Geometry check sheet. Reference: the model listing, model coordinates, mm. A direction names the side the tool comes from. Round coordinates to 2 decimals unless told otherwise and drop trailing zeros. Write each loop counter-clockwise with the first axis right and the second up, starting at its lowest first coordinate (ties: lowest second). Pieces come first, ordered by that corner, then holes. Notation, with made-up numbers: M 16.5,36 L 39.5,36 A34 cw 39.5,68 Z; hole C -28.75,80 d4. An arc over 180 degrees is marked long. Answer in a Markdown table with one row per item. Add a question column.
from build123d import *

# Parameters (mm, degrees)
SKETCH1_R                 = 1.778
BOSS_EXTRUDE1_DEPTH       = 6.35
FILLET1_R                 = 1.27
F_6_32_TAPPED_HOLE1_D     = 2.7051
F_6_CLEARANCE_HOLE1_D     = 3.6576
F_6_CLEARANCE_HOLE1_DEPTH = 3.175
F_6_CLEARANCE_HOLE1_TIP   = 1.0988539


with BuildPart() as part:
    # Sketch1 → Boss-Extrude1 (new body)
    with BuildSketch(Plane.XY):
        with BuildLine():
            Line((-5.04, 40.467867395), (-5.04, 31.75))
            Line((-5.04, 31.75), (-5.04, 5.617641854))
            ThreePointArc((-5.04, 5.617641854), (-5.205917611, 4.175551358), (-5.695, 2.808820927))
            ThreePointArc((-5.695, 2.808820927), (1.46358213, -6.179031263), (3.83, 5.064938302))
            ThreePointArc((3.83, 5.064938302), (1.974799916, 7.301272707), (1.31, 10.129876603))
            Line((1.31, 10.129876603), (1.31, 23.320498235))
            ThreePointArc((1.31, 23.320498235), (1.853099889, 25.890013969), (3.389499561, 28.020000975))
            ThreePointArc((3.389499561, 28.020000975), (4.60894119, 29.710573339), (5.04, 31.75))
            Line((5.04, 31.75), (5.04, 40.467867395))
            Line((5.04, 40.467867395), (2.5, 40.467867395))
            Line((2.5, 40.467867395), (2.5, 31.75))
            ThreePointArc((2.5, 31.75), (-1.456880228, 29.718375035), (-0.802, 34.117867395))
            Line((-0.802, 34.117867395), (-0.802, 40.467867395))
            Line((-0.802, 40.467867395), (-5.04, 40.467867395))
        make_face()
        Circle(SKETCH1_R, mode=Mode.SUBTRACT)
    extrude(amount=BOSS_EXTRUDE1_DEPTH)

    # Fillet1
    fillet1_edges = [part.edges().sort_by_distance(p)[0] for p in [
        (-5.04, 40.467867395, 3.175),
    ]]
    fillet(fillet1_edges, radius=FILLET1_R)

    # #6-32 Tapped Hole1 (through all)
    with Locations(Plane.ZY.offset(5.04)):
        with Locations((3.175, 37.292867395)):
            Hole(F_6_32_TAPPED_HOLE1_D / 2)

    # #6 Clearance Hole1
    with Locations(Plane(origin=(5.04, 37.292867395, 3.175), x_dir=(0, 1, 0), z_dir=(1, 0, 0))):
        with Locations((0, 0)):
            Hole(F_6_CLEARANCE_HOLE1_D / 2, depth=F_6_CLEARANCE_HOLE1_DEPTH)
            with Locations((0, 0, -(F_6_CLEARANCE_HOLE1_DEPTH + F_6_CLEARANCE_HOLE1_TIP / 2))):  # 118° drill point
                Cone(0, F_6_CLEARANCE_HOLE1_D / 2, F_6_CLEARANCE_HOLE1_TIP, mode=Mode.SUBTRACT)


solid = part.part
Item 1: Gauge pin test, flat ends, axial feed: pin 1 Ø3 at (y, z) = (38.5, 3.5) entering from +X; pin 2 Ø2 at (y, z) = (34, 4) entering from -X; pin 3 Ø3 at (x, y) = (0, 0) entering from -Z. Record the tip position at first contact, or that the pin passes through.
Item 2: Scan lines: probe 1 along X at (y, z) = (31.75, 2); probe 2 along Y at (x, z) = (0, 1.5); probe 3 along Y at (x, z) = (-1, 2.75). Record each from-to range of solid material in increasing order. Write a range as from..to.
Item 3: Section check D-D, the plane y = 17. Record the boundary of the cut face in (x, z).
Item 4: Mould release check, pull along Y, two halves, no side actions. Record for faces 6 (the cylindrical face through (4.597, 29.684, 3.131)), 7 (the cylindrical face through (-4.678, 40.086, 3.219)), 8 (the flat face through (5.04, 35, 3)): +Y half, -Y half, draft (parallel to the pull), parting line (faces both ways), or undercut.
Item 5: Section check A-A, the plane y = 0. Record the boundary of the cut face in (x, z).
Item 6: Access from +Z, -Z, +X, -X, +Y, -Y to the whole of each face (thin tool, end or side, straight path). Record for faces 1 (the flat face through (-2, 17, 0)), 2 (the cylindrical face through (3.75, 39.12, 3.26)), 3 (the flat face through (1.31, 17, 3)), 4 (the flat face through (-5.04, 23, 3)), 5 (the flat face through (2.5, 35, 3)).
Item 7: Section check B-B, the plane x = 0. Record the boundary of the cut face in (y, z).
Item 8: Section check C-C, the plane z = 4. Give the number of separate pieces and of enclosed holes in the cut face, and give its area (3 significant figures).
Result sheet:
| question | item | result |
|---|---|---|
| 1 | pin 1 | stops at x = 5.04 |
| 1 | pin 2 | stops at x = -5.04 |
| 1 | pin 3 | passes through |
| 2 | probe 1 | x = -5.04..-2.5, 2.5..5.04 |
| 2 | probe 2 | y = -6.35..-1.78, 1.78..29.25 |
| 2 | probe 3 | y = -6.27..-1.47, 1.47..29.46, 34.04..36.01, 38.58..40.47 |
| 3 | outline | M -5.04,0 L 1.31,0 L 1.31,6.35 L -5.04,6.35 Z |
| 4 | face 6 | undercut |
| 4 | face 7 | +Y half |
| 4 | face 8 | draft |
| 5 | outline | M -6.35,0 L -1.78,0 L -1.78,6.35 L -6.35,6.35 Z; M 1.78,0 L 6.35,0 L 6.35,6.35 L 1.78,6.35 Z |
| 6 | face 1 | -Z, +X, -X, +Y, -Y |
| 6 | face 2 | +X |
| 6 | face 3 | +Z, -Z, +X |
| 6 | face 4 | +Z, -Z, -X, +Y |
| 6 | face 5 | +Z, -Z, +Y |
| 7 | outline | M -6.35,0 L -1.78,0 L -1.78,6.35 L -6.35,6.35 Z; M 1.78,0 L 29.25,0 L 29.25,6.35 L 1.78,6.35 Z |
| 8 | separate pieces | 3 |
| 8 | enclosed holes | 1 |
| 8 | area | 328 mm^2 |
